Job drawing, mm, ordinate dimensions from the low corner. One solid piece. A direction names the side the tool comes from. Give positions to 0.01 mm unless a question says otherwise; leave off trailing zeros. Loops run counter-clockwise (first coordinate to the right, second up) from the corner with the lowest first, then second, coordinate; pieces in that order, holes last.
Item 1: Drop flat-ended pins along their axis: P1, Ø9, axis at y = 6.5, z = 18, coming from the +X side; P2, Ø5.5, axis at x = 12.5, z = 22, coming from the -Y side; P3, Ø14.5, axis at x = 7.5, y = 10, coming from the +Z side. Give the stop position or say it passes through.
Item 2: Saw through at C-C on z = 19. Give the cut face in (x, y), plus the area to 3 significant figures.
Item 3: Probe probe 1 along Y at (x, z) = (34.5, 30.5); probe 2 along Z at (x, y) = (15, 7); probe 3 along Z at (x, y) = (26.5, 8.5). List the from-to ranges inside material, lowest first.
Item 4: Saw through at B-B on x = 23. Give the cut face in (y, z), plus the area to 3 significant figures.
Item 5: Saw through at A-A on y = 20. Give the cut face in (x, z).
Item 6: Saw through at D-D on x = 43. Give the cut face in (y, z), plus the area to 3 significant figures.
Item 7: Which spindle directions (+Z, -Z, +X, -X, +Y, -Y) get a long thin tool onto all of the face, cutting with end or side? Do the marked faces 1, 2 and 3. Say none if no direction does.
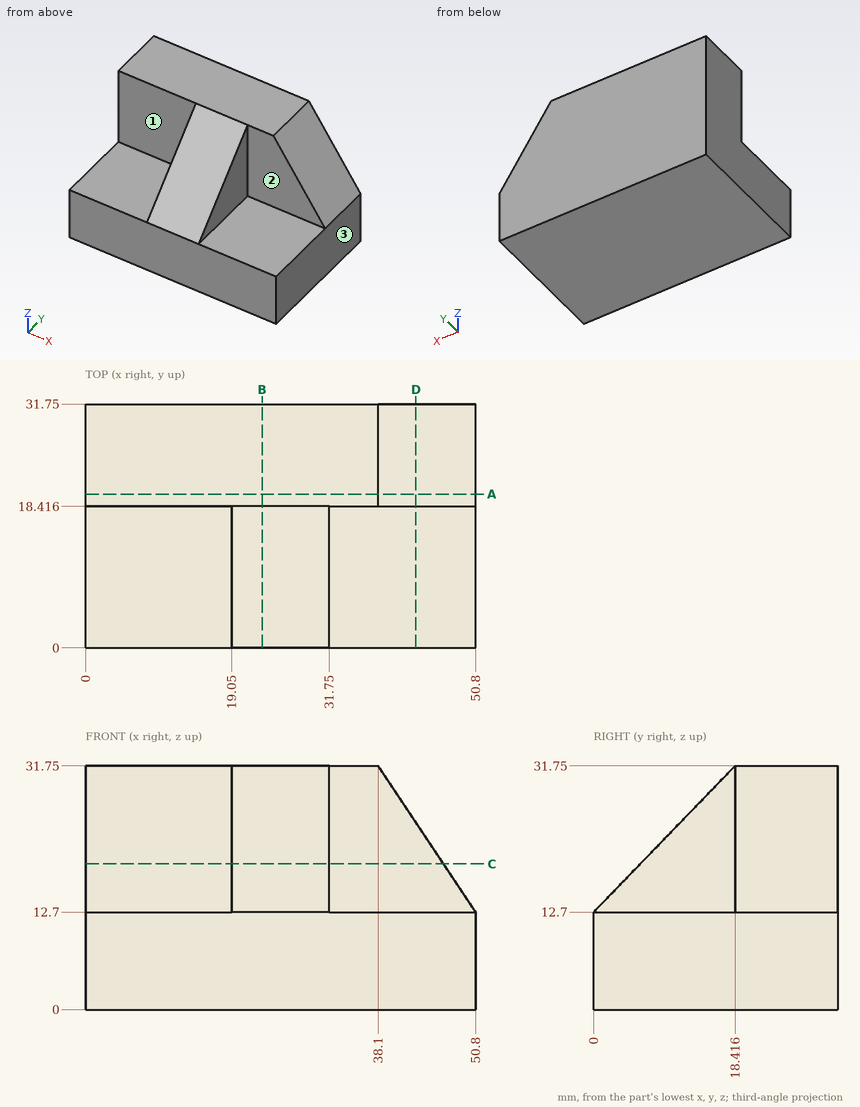
Results below:
1. P1: stops at x = 31.75
1. P2: stops at y = 18.42
1. P3: stops at z = 12.7
2. outline: (0, 18.42) - (19.05, 18.42) - (19.05, 6.09) - (31.75, 6.09) - (31.75, 18.42) - (46.6, 18.42) - (46.6, 31.75) - (0, 31.75) - close
2. area: 778 mm2
3. probe 1: y = 18.42 to 31.75
3. probe 2: z = 0 to 12.7
3. probe 3: z = 0 to 21.49
4. outline: (0, 0) - (31.75, 0) - (31.75, 31.75) - (18.42, 31.75) - (0, 12.7) - close
4. area: 833 mm2
5. outline: (0, 0) - (50.8, 0) - (50.8, 12.7) - (38.1, 31.75) - (0, 31.75) - close
6. outline: (0, 0) - (31.75, 0) - (31.75, 24.4) - (18.42, 24.4) - (18.42, 12.7) - (0, 12.7) - close
6. area: 559 mm2
7. face 1: +Z, -X, -Y
7. face 2: +Z, +X, -Y
7. face 3: +Z, -Z, +X, +Y, -Y
